Design review of the part built by this model. Coordinates are the model's own, in mm. Face numbers are marked on the shaded views. Round coordinates to 2 decimals unless told otherwise and drop trailing zeros. Loops run counter-clockwise (first coordinate to the right, second up) from the corner with the lowest first, then second, coordinate; pieces in that order, holes last. Notation, with made-up numbers: (49, 24.5) - (101, 24.5) arc R11 ccw to (101, 29.5) - close; hole circle Ø6 at (54.5, -35.5). An arc over 180 degrees is marked (long way). Return JSON: item names as keys, results as strings. Group by question number.
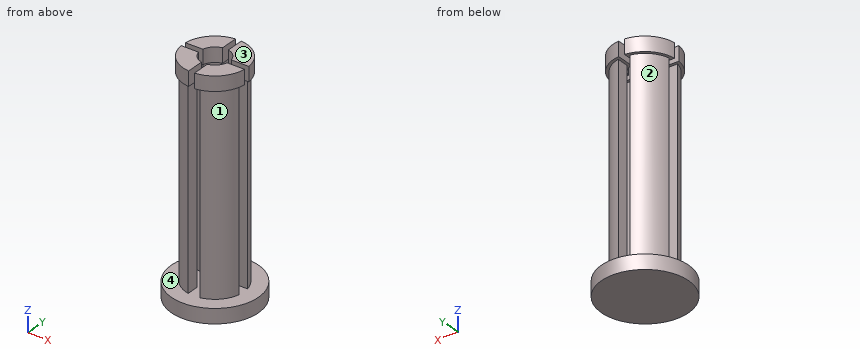
from build123d import *

# Parameters (mm, degrees)
SKETCH1_R           = 2
BOSS_EXTRUDE1_DEPTH = 13.5
SKETCH2_R           = 1.2
CUT_EXTRUDE1_DEPTH  = 14.793114224
SKETCH3_W           = 0.8
SKETCH3_H           = 6.59267807
SKETCH3_W_2         = 7.006923124
SKETCH3_H_2         = 0.8
CUT_EXTRUDE3_DEPTH  = 14.793114224
BOSS_EXTRUDE2_DEPTH = 1
SKETCH5_R           = 3
BOSS_EXTRUDE3_DEPTH = 1


with BuildPart() as part:
    # Sketch1 → Boss-Extrude1 (new body)
    with BuildSketch(Plane.XY):
        Circle(SKETCH1_R)
    extrude(amount=BOSS_EXTRUDE1_DEPTH)

    # Sketch2 → Cut-Extrude1 (cut, through all)
    with BuildSketch(Plane.XY.offset(13.5)):
        Circle(SKETCH2_R)
    extrude(amount=-CUT_EXTRUDE1_DEPTH, mode=Mode.SUBTRACT)

    # Sketch3 → Cut-Extrude3 (cut, through all)
    with BuildSketch(Plane.XY.offset(13.5)):
        Rectangle(SKETCH3_W, SKETCH3_H)
        Rectangle(SKETCH3_W_2, SKETCH3_H_2)
    extrude(amount=-CUT_EXTRUDE3_DEPTH, mode=Mode.SUBTRACT)


with BuildPart() as cut_extrude3_piece_1:
    # of the separate pieces the step leaves, piece 1, a body of its own (cut_extrude3_pieces)
    add(part.part.solids().sort_by_distance((1.959591794, 0.4, 0))[0])



with BuildPart() as cut_extrude3_piece_2:
    # of the separate pieces the step leaves, piece 2, a body of its own (cut_extrude3_pieces)
    add(part.part.solids().sort_by_distance((0.4, -1.959591794, 0))[0])


with BuildPart() as cut_extrude3_piece_3:
    # of the separate pieces the step leaves, piece 3, a body of its own (cut_extrude3_pieces)
    add(part.part.solids().sort_by_distance((-1.959591794, -0.4, 0))[0])


with BuildPart() as cut_extrude3_piece_4:
    # of the separate pieces the step leaves, piece 4, a body of its own (cut_extrude3_pieces)
    add(part.part.solids().sort_by_distance((-0.4, 1.959591794, 0))[0])


with BuildPart() as cut_extrude3_piece_1_1:
    add(cut_extrude3_piece_1.part)

    add(cut_extrude3_piece_2.part)  # Boss-Extrude2 merges Cut-Extrude3 piece 2

    add(cut_extrude3_piece_3.part)  # Boss-Extrude2 merges Cut-Extrude3 piece 3

    add(cut_extrude3_piece_4.part)  # Boss-Extrude2 merges Cut-Extrude3 piece 4
    # Sketch4 → Boss-Extrude2 (add)
    with BuildSketch(Plane.XY.offset(13.5)):
        with BuildLine():
            Line((-2.19089023, 0.2), (-0.979795897, 0.2))
            ThreePointArc((-0.979795897, 0.2), (-0.707106781, 0.707106781), (-0.2, 0.979795897))
            Line((-0.2, 0.979795897), (-0.2, 2.19089023))
            ThreePointArc((-0.2, 2.19089023), (-1.555634919, 1.555634919), (-2.19089023, 0.2))
        make_face()
        with BuildLine():
            Line((0.979795897, 0.2), (2.19089023, 0.2))
            ThreePointArc((2.19089023, 0.2), (1.555634919, 1.555634919), (0.2, 2.19089023))
            Line((0.2, 2.19089023), (0.2, 0.979795897))
            ThreePointArc((0.2, 0.979795897), (0.707106781, 0.707106781), (0.979795897, 0.2))
        make_face()
        with BuildLine():
            Line((0.2, -0.979795897), (0.2, -2.19089023))
            ThreePointArc((0.2, -2.19089023), (1.555634919, -1.555634919), (2.19089023, -0.2))
            Line((2.19089023, -0.2), (0.979795897, -0.2))
            ThreePointArc((0.979795897, -0.2), (0.707106781, -0.707106781), (0.2, -0.979795897))
        make_face()
        with BuildLine():
            Line((-0.979795897, -0.2), (-2.19089023, -0.2))
            ThreePointArc((-2.19089023, -0.2), (-1.555634919, -1.555634919), (-0.2, -2.19089023))
            Line((-0.2, -2.19089023), (-0.2, -0.979795897))
            ThreePointArc((-0.2, -0.979795897), (-0.707106781, -0.707106781), (-0.979795897, -0.2))
        make_face()
    extrude(amount=BOSS_EXTRUDE2_DEPTH)

    # Sketch5 → Boss-Extrude3 (add)
    with BuildSketch(Plane(origin=(0, 0, 0), x_dir=(-1, 0, 0), z_dir=(0, 0, -1))):
        Circle(SKETCH5_R)
    extrude(amount=BOSS_EXTRUDE3_DEPTH)


solid = cut_extrude3_piece_1_1.part
Q1. Add section B-B, the plane x = -1.7. State the section outline as (y, z) points.
Q2. For line 1 (X direction, y = 1.65, z = 12.75); line 2 (X direction, y = 0.65, z = 1); line 3 (Y direction, x = 1.7, z = 8), list the stretches that pass through material, from the lowest coordinate up.
Q3. Add section D-D, the plane y = -1.5. State the section outline as (x, z) points, plus the area to 3 significant figures.
Q4. Draft analysis for pull direction Y (two halves, no side actions). For the marked faces 1, 2, 3 and 4, state which applies: pulls with the +Y half, pulls with the -Y half, needs draft (parallel to the pull), parting line crosses it, or undercut.
Q5. Add section C-C, the plane y = 0. State the section outline as (x, z) points.
Q6. Insertion check: pin 1 Ø1.1 at (y, z) = (1.5, 14) entering from +X; pin 2 Ø0.8 at (x, z) = (-2, 14) entering from +Y; pin 3 Ø0.8 at (y, z) = (1.5, 14) entering from -X. Each pin has a flat end and moves straight along its axis. Give the tip position at first contact, or say it passes through.
Q7. Add section A-A, the plane z = 9.5. State the section outline as (x, y) points, plus the area to 3 significant figures.
Evaluation:
{
 "1": {"outline": "(-2.47, -1) - (2.47, -1) - (2.47, 0) - (1.05, 0) - (1.05, 13.5) - (1.4, 13.5) - (1.4, 14.5) - (0.2, 14.5) - (0.2, 13.5) - (0.4, 13.5) - (0.4, 0) - (-0.4, 0) - (-0.4, 13.5) - (-0.2, 13.5) - (-0.2, 14.5) - (-1.4, 14.5) - (-1.4, 13.5) - (-1.05, 13.5) - (-1.05, 0) - (-2.47, 0) - close"},
 "2": {"line 1": "-1.13 to -0.4, 0.4 to 1.13", "line 2": "-1.89 to -1.01, 1.01 to 1.89", "line 3": "-1.05 to -0.4, 0.4 to 1.05"},
 "3": {"outline": "(-2.6, -1) - (2.6, -1) - (2.6, 0) - (1.32, 0) - (1.32, 13.5) - (1.61, 13.5) - (1.61, 14.5) - (0.2, 14.5) - (0.2, 13.5) - (0.4, 13.5) - (0.4, 0) - (-0.4, 0) - (-0.4, 13.5) - (-0.2, 13.5) - (-0.2, 14.5) - (-1.61, 14.5) - (-1.61, 13.5) - (-1.32, 13.5) - (-1.32, 0) - (-2.6, 0) - close", "area": "32.9 mm²"},
 "4": {"face 1": "pulls with the -Y half", "face 2": "pulls with the +Y half", "face 3": "needs draft", "face 4": "undercut"},
 "5": {"outline": "(-3, -1) - (3, -1) - (3, 0) - (-3, 0) - close"},
 "6": {"pin 1": "x = 1.98", "pin 2": "y = 1.51", "pin 3": "x = -1.91"},
 "7": {"outline": "(-1.96, -0.4) arc R2 ccw to (-0.4, -1.96) - (-0.4, -1.13) arc R1.2 cw to (-1.13, -0.4) - close; (-1.96, 0.4) - (-1.13, 0.4) arc R1.2 cw to (-0.4, 1.13) - (-0.4, 1.96) arc R2 ccw to start; (0.4, -1.96) arc R2 ccw to (1.96, -0.4) - (1.13, -0.4) arc R1.2 cw to (0.4, -1.13) - close; (0.4, 1.13) arc R1.2 cw to (1.13, 0.4) - (1.96, 0.4) arc R2 ccw to (0.4, 1.96) - close", "area": "5.45 mm²"}
}
